Check sheet for the modelled part. Datum: model origin and axes. Units: mm. Face numbers are marked on the shaded views. Coordinates: 2 decimals unless noted, no trailing zeros. Loops run counter-clockwise (first coordinate to the right, second up) from the corner with the lowest first, then second, coordinate; pieces in that order, holes last. Notation, with made-up numbers: M -40,-7.5 L -5,-7.5 A34 ccw -5,24.5 Z; hole C 47,76.25 d9. An arc over 180 degrees is marked long. Return JSON: item names as keys, results as strings.
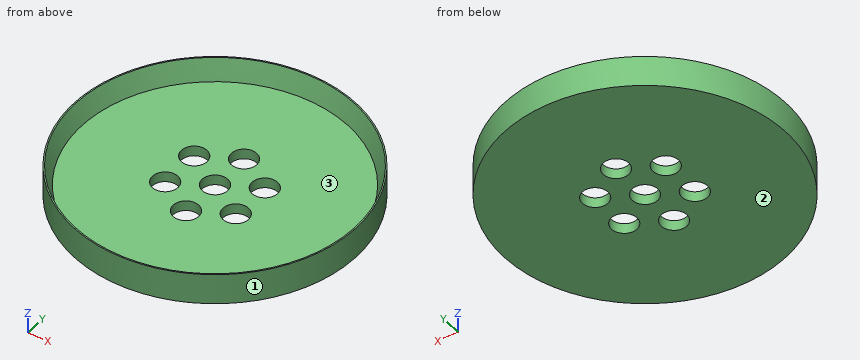
from build123d import *

# Parameters (mm, degrees)
F0_R     = 26
F0_R_2   = 12
F0_R_3   = 2.5
F1_DEPTH = 2
F0_R_4   = 27.5
F2_DEPTH = 6
F3_SIZE2 = 1.24999
F3_SIZE  = 3.99999


# Not quite as in the source:
# - a fillet or chamfer is up to 0.001 mm smaller than in the source, because OpenCascade refuses the exact size


with BuildPart() as f1:
    # F0 (on Top) → F1 (new body)
    with BuildSketch(Plane.XY):
        Circle(F0_R)
        Circle(F0_R_2, mode=Mode.SUBTRACT)
        Circle(F0_R_2)
        with Locations((-6.9282032303, -4)):
            Circle(F0_R_3, mode=Mode.SUBTRACT)
        with Locations((0, -8)):
            Circle(F0_R_3, mode=Mode.SUBTRACT)
        with Locations((6.9282032303, -4)):
            Circle(F0_R_3, mode=Mode.SUBTRACT)
        with Locations((-6.9282032303, 4)):
            Circle(F0_R_3, mode=Mode.SUBTRACT)
        Circle(F0_R_3, mode=Mode.SUBTRACT)
        with Locations((6.9282032303, 4)):
            Circle(F0_R_3, mode=Mode.SUBTRACT)
        with Locations((0, 8)):
            Circle(F0_R_3, mode=Mode.SUBTRACT)
    extrude(amount=F1_DEPTH)

    # F0 (on Top) → F2 (join)
    with BuildSketch(Plane.XY):
        Circle(F0_R_4)
        Circle(F0_R, mode=Mode.SUBTRACT)
    extrude(amount=F2_DEPTH)

    # F3 (size 4 and 1.25 in the source; OpenCascade refuses exactly that, so slightly less here)
    f3_edges = [f1.edges().sort_by_distance(p)[0] for p in [
        (-26, 0, 6),
    ]]
    f3_side = f1.faces().sort_by_distance((-26, 0, 4))[0]
    chamfer(f3_edges, length=F3_SIZE, length2=F3_SIZE2, reference=f3_side)


solid = f1.part
1) Draft check along Y on the marked faces 1, 2 and 3. Enter one of: +Y half, -Y half, draft (parallel to the pull), parting line (faces both ways), or undercut.
Answers:
{"face 1": "parting line", "face 2": "draft", "face 3": "undercut"}
2) Scan lines: line 1 along Y through (x, z) = (0, 0.7); line 2 along Y through (x, z) = (-1.5, 1.4); line 3 along Z through (x, y) = (1.5, 13.5). Record each from-to range of solid material in increasing order. Write a range as [from, to].
Answers:
{"line 1": "[-27.5, -10.5], [-5.5, -2.5], [2.5, 5.5], [10.5, 27.5]", "line 2": "[-27.46, -10], [-6, -2], [2, 6], [10, 27.46]", "line 3": "[0, 2]"}
3) Go/stop test with flat-tipped pins: pin 1 Ø1 at (y, z) = (8, 5) entering from +X; pin 2 Ø1.5 at (x, z) = (8, 0.5) entering from +Y; pin 3 Ø3 at (x, y) = (1.5, -12.5) entering from +Z. Record where each tip stops, or that it passes through.
Answers:
{"pin 1": "x = 26.46", "pin 2": "y = 26.53", "pin 3": "z = 2"}
4) Section check C-C on z = 5.15. Record the cut outline in (x, y).
Answers:
{"outline": "C 0,0 d55; hole C 0,0 d53.97"}
5) Section check A-A on x = 0. Count the separate pieces of the cut face and the enclosed holes in it, then the cut area to 3 significant figures.
Answers:
{"separate pieces": "4", "enclosed holes": "0", "area": "87.0 mm²"}
6) Section check B-B on z = 0.8. Record the cut outline in (x, y), then the cut area to 3 significant figures.
Answers:
{"outline": "C 0,0 d55; hole C -6.93,-4 d5; hole C -6.93,4 d5; hole C 0,-8 d5; hole C 0,0 d5; hole C 0,8 d5; hole C 6.93,-4 d5; hole C 6.93,4 d5", "area": "2,240 mm²"}
